from build123d import *

# Parameters (mm, degrees)
SKETCH1_R           = 1.6
SKETCH1_R_2         = 1.1
SKETCH1_R_3         = 1.75
SKETCH1_R_4         = 6.1
SKETCH1_W           = 10
SKETCH1_H           = 3
BOSS_EXTRUDE1_DEPTH = 3
FILLET1_R           = 5


with BuildPart() as part:
    # Sketch1 → Boss-Extrude1 (new body)
    with BuildSketch(Plane(origin=(0, 0, 0), x_dir=(1, 0, 0), z_dir=(0, 1, 0))):
        with BuildLine():
            Line((40, 87.5), (40, 57.5))
            Line((40, 57.5), (120, 57.5))
            Line((120, 57.5), (120, 87.5))
            Line((120, 87.5), (136.956007081, 87.5))
            ThreePointArc((136.956007081, 87.5), (150, 0), (136.956007081, -87.5))
            Line((136.956007081, -87.5), (120, -87.5))
            Line((120, -87.5), (120, -57.5))
            Line((120, -57.5), (40, -57.5))
            Line((40, -57.5), (40, -87.5))
            Line((40, -87.5), (-19.054445662, -87.5))
            Line((-19.054445662, -87.5), (-19.054445662, -77.5))
            Line((-19.054445662, -77.5), (-9.054445662, -67.5))
            Line((-9.054445662, -67.5), (-9.054445662, -57.465130862))
            Line((-9.054445662, -57.465130862), (-29.037011093, -37.482565431))
            Line((-29.037011093, -37.482565431), (-56.537011093, -37.482565431))
            Line((-56.537011093, -37.482565431), (-56.537011093, -50))
            Line((-56.537011093, -50), (-66.537011093, -50))
            Line((-66.537011093, -50), (-66.537011093, -37.482565431))
            Line((-66.537011093, -37.482565431), (-94.037011093, -37.482565431))
            Line((-94.037011093, -37.482565431), (-114.054445662, -57.5))
            Line((-114.054445662, -57.5), (-114.054445662, -67.5))
            Line((-114.054445662, -67.5), (-104.054445662, -77.5))
            Line((-104.054445662, -77.5), (-104.054445662, -87.5))
            Line((-104.054445662, -87.5), (-126.554445662, -87.5))
            ThreePointArc((-126.554445662, -87.5), (-150, 0), (-126.554445662, 87.5))
            Line((-126.554445662, 87.5), (-104.054445662, 87.5))
            Line((-104.054445662, 87.5), (-104.054445662, 77.5))
            Line((-104.054445662, 77.5), (-114.054445662, 67.5))
            Line((-114.054445662, 67.5), (-114.054445662, 57.5))
            Line((-114.054445662, 57.5), (-94.037011093, 37.482565431))
            Line((-94.037011093, 37.482565431), (-66.537011093, 37.482565431))
            Line((-66.537011093, 37.482565431), (-66.537011093, 50))
            Line((-66.537011093, 50), (-56.537011093, 50))
            Line((-56.537011093, 50), (-56.537011093, 37.482565431))
            Line((-56.537011093, 37.482565431), (-29.037011093, 37.482565431))
            Line((-29.037011093, 37.482565431), (-9.054445662, 57.465130862))
            Line((-9.054445662, 57.465130862), (-9.054445662, 67.5))
            Line((-9.054445662, 67.5), (-19.054445662, 77.5))
            Line((-19.054445662, 77.5), (-19.054445662, 87.5))
            Line((-19.054445662, 87.5), (40, 87.5))
        make_face()
        with Locations(Location((-120, -40, 0), (0, 0, 270))):
            Circle(SKETCH1_R, mode=Mode.SUBTRACT)
        with Locations(Location((0, -40, 0), (0, 0, 270))):
            Circle(SKETCH1_R, mode=Mode.SUBTRACT)
        with Locations(Location((120, -40, 0), (0, 0, 270))):
            Circle(SKETCH1_R, mode=Mode.SUBTRACT)
        with Locations(Location((120, 40, 0), (0, 0, 90))):
            Circle(SKETCH1_R, mode=Mode.SUBTRACT)
        with Locations(Location((0, 40, 0), (0, 0, 90))):
            Circle(SKETCH1_R, mode=Mode.SUBTRACT)
        with Locations(Location((-120, 40, 0), (0, 0, 90))):
            Circle(SKETCH1_R, mode=Mode.SUBTRACT)
        with Locations(Location((-15, 21, 0), (0, 0, 270))):
            Circle(SKETCH1_R, mode=Mode.SUBTRACT)
        with Locations(Location((9, 21, 0), (0, 0, 270))):
            Circle(SKETCH1_R, mode=Mode.SUBTRACT)
        with Locations(Location((9, -21, 0), (0, 0, 90))):
            Circle(SKETCH1_R, mode=Mode.SUBTRACT)
        with Locations(Location((-15, -21, 0), (0, 0, 90))):
            Circle(SKETCH1_R, mode=Mode.SUBTRACT)
        with Locations(Location((123.8, 13.4, 0), (0, 0, 270))):
            Circle(SKETCH1_R_2, mode=Mode.SUBTRACT)
        with Locations(Location((65, 13.4, 0), (0, 0, 270))):
            Circle(SKETCH1_R_2, mode=Mode.SUBTRACT)
        with Locations(Location((65, -13.4, 0), (0, 0, 90))):
            Circle(SKETCH1_R_2, mode=Mode.SUBTRACT)
        with Locations(Location((123.8, -13.4, 0), (0, 0, 90))):
            Circle(SKETCH1_R_2, mode=Mode.SUBTRACT)
        with Locations(Location((-61.537011093, -45, 0), (0, 0, 270))):
            Circle(SKETCH1_R_3, mode=Mode.SUBTRACT)
        with Locations(Location((-61.537011093, 45, 0), (0, 0, 90))):
            Circle(SKETCH1_R_3, mode=Mode.SUBTRACT)
        with Locations(Location((-61.537011093, -10, 0), (0, 0, 270))):
            Circle(SKETCH1_R, mode=Mode.SUBTRACT)
        with Locations(Location((-61.537011093, 10, 0), (0, 0, 90))):
            Circle(SKETCH1_R, mode=Mode.SUBTRACT)
        with Locations(Location((36, 0, 0), (0, 0, 270))):
            Circle(SKETCH1_R_4, mode=Mode.SUBTRACT)
        with Locations((59.4, 36.4)):
            Rectangle(SKETCH1_W, SKETCH1_H, mode=Mode.SUBTRACT)
        with Locations((59.4, -36.4)):
            Rectangle(SKETCH1_W, SKETCH1_H, mode=Mode.SUBTRACT)
    extrude(amount=BOSS_EXTRUDE1_DEPTH)

    # Fillet1
    fillet1_edges = [part.edges().sort_by_distance(p)[0] for p in [
        (-104.054445662, 1.5, -87.5),
        (-104.054445662, 1.5, -77.5),
        (-114.054445662, 1.5, -67.5),
        (-114.054445662, 1.5, -57.5),
        (-9.054445662, 1.5, -57.465130862),
        (-9.054445662, 1.5, -67.5),
        (-19.054445662, 1.5, -77.5),
        (-19.054445662, 1.5, -87.5),
        (40, 1.5, -87.5),
        (40, 1.5, -57.5),
        (120, 1.5, -57.5),
        (120, 1.5, -87.5),
        (136.956007081, 1.5, -87.5),
        (136.956007081, 1.5, 87.5),
        (120, 1.5, 87.5),
        (120, 1.5, 57.5),
        (40, 1.5, 57.5),
        (40, 1.5, 87.5),
        (-19.054445662, 1.5, 87.5),
        (-19.054445662, 1.5, 77.5),
        (-9.054445662, 1.5, 67.5),
        (-9.054445662, 1.5, 57.465130862),
        (-114.054445662, 1.5, 57.5),
        (-114.054445662, 1.5, 67.5),
        (-104.054445662, 1.5, 77.5),
        (-104.054445662, 1.5, 87.5),
        (-126.554445662, 1.5, 87.5),
        (-126.554445662, 1.5, -87.5),
        (-56.537011093, 1.5, -50),
        (-94.037011093, 1.5, -37.482565431),
        (-29.037011093, 1.5, -37.482565431),
        (-66.537011093, 1.5, -50),
        (-29.037011093, 1.5, 37.482565431),
        (-94.037011093, 1.5, 37.482565431),
        (-56.537011093, 1.5, 50),
        (-66.537011093, 1.5, 50),
        (-66.537011093, 1.5, -37.482565431),
        (-56.537011093, 1.5, -37.482565431),
        (-66.537011093, 1.5, 37.482565431),
        (-56.537011093, 1.5, 37.482565431),
    ]]
    fillet(fillet1_edges, radius=FILLET1_R - 0.0001)  # a hair under: the kernel refuses the full size


solid = part.part
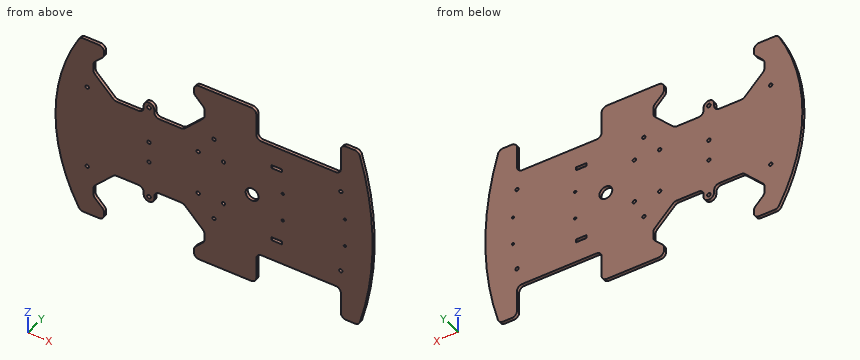
Model file for the job. Use its own axes, mm. Round coordinates to 2 decimals unless told otherwise and drop trailing zeros. Loops run counter-clockwise (first coordinate to the right, second up) from the corner with the lowest first, then second, coordinate; pieces in that order, holes last. Notation, with made-up numbers: M -30.75,-25 L 5.25,-25 A23 cw 5.25,-13 Z; hole C 49.25,-14.75 d11. An arc over 180 degrees is marked long. One line per question, with ' | ' between items.
1) Band-saw the part on A-A (z = -53). Give the cut face in (x, y), then the cut area to 3 significant figures.
Solved:
outline: M -141.78,0 L -109.55,0 L -109.55,3 L -141.78,3 Z; M -13.52,0 L 145.28,0 L 145.28,3 L -13.52,3 Z | area: 573 mm²
2) Band-saw the part on B-B (x = -37.5). Give the cut face in (y, z).
Solved:
outline: M 0,-37.48 L 3,-37.48 L 3,37.48 L 0,37.48 Z
3) Drill centre lines: line 1 along Z through (x, y) = (-120, 1.4); line 2 along Z through (x, y) = (65, 1.5); line 3 along X through (y, z) = (2.1, 13.4). Where is each one in solid material? Low to high.
Solved:
line 1: z = -87.5 to -41.6, -38.4 to 38.4, 41.6 to 87.5 | line 2: z = -57.5 to -14.5, -12.3 to 12.3, 14.5 to 57.5 | line 3: x = -149.49 to 63.9, 66.1 to 122.7, 124.9 to 149.7
4) Flat gauge pins, fed straight in: pin 1 (0.8 mm diameter, centred on y = 1.5, z = 44, fed in from -X); pin 2 (0.9 mm diameter, centred on y = 2, z = 36.5, fed in from -X); pin 3 (1 mm diameter, centred on y = 0.5, z = -55.5, fed in from +X). Where does each tip first touch, or does it go through?
Solved:
pin 1: stops at x = -144.48 | pin 2: stops at x = -146.25 | pin 3: stops at x = 144.92
5) Band-saw the part on C-C (y = 1.6). Give the number of separate pieces and of enclosed holes in the cut face, then the cut area to 3 significant figures.
Solved:
separate pieces: 1 | enclosed holes: 21 | area: 36,400 mm²
6) Band-saw the part on D-D (x = 85). Give the cut face in (y, z).
Solved:
outline: M 0,-57.5 L 3,-57.5 L 3,57.5 L 0,57.5 Z
